Geometry check sheet. Reference: drawing and pictorial views, mm from the part's lowest x, y, z. A direction names the side the tool comes from. Coordinates: 2 decimals unless noted, no trailing zeros. Write each loop counter-clockwise with the first axis right and the second up, starting at its lowest first coordinate (ties: lowest second). Pieces come first, ordered by that corner, then holes. Notation, with made-up numbers: (11.5, 63.25) -> (55.5, 63.25) arc R34 cw to (55.5, 102.25) -> close; hole circle Ø5 at (-39, 69.5). An arc over 180 degrees is marked (long way). Answer in a Markdown table with one row per item.
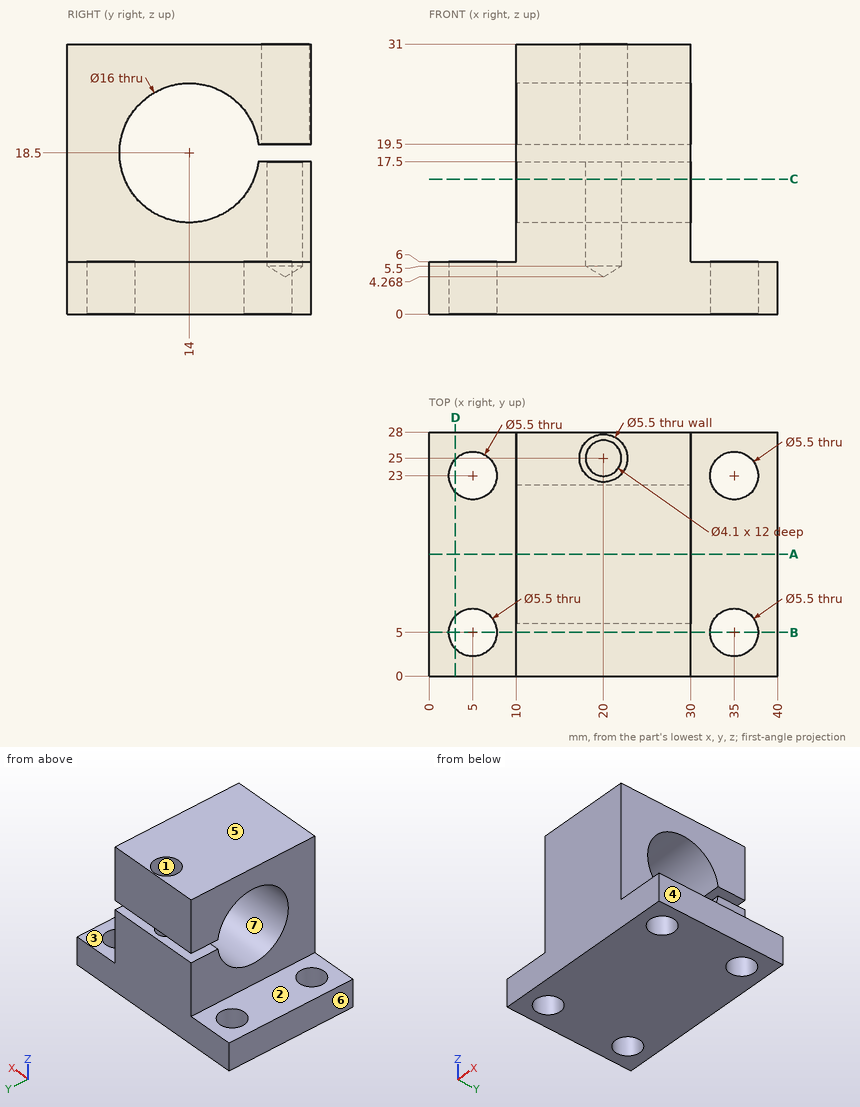
1. Section check C-C, the plane z = 15.5. Record the boundary of the cut face in (x, y), plus the area to 3 significant figures.
Geometry says:
| item | result |
|---|---|
| outline | (10, 0) -> (30, 0) -> (30, 6.58) -> (10, 6.58) -> close; (10, 21.42) -> (30, 21.42) -> (30, 28) -> (10, 28) -> close; hole circle Ø4.1 at (20, 25) |
| area | 250 mm^2 |
2. Tool access check on the marked faces 1, 2, 3 and 4. Record the directions out of +Z, -Z, +X, -X, +Y, -Y that give a thin tool (end or side, any length) a straight path to the whole face; none if there is none.
Geometry says:
| item | result |
|---|---|
| face 1 | +Z |
| face 2 | +Z, -X, +Y, -Y |
| face 3 | +Z, +X, +Y, -Y |
| face 4 | +Z, -Z, +X, +Y, -Y |
3. Depth check by flat-ended pin: P1, Ø6.5, axis at x = 35, y = 5, coming from the +Z side; P2, Ø12, axis at y = 23, z = 20.5, coming from the +X side; P3, Ø4.5, axis at x = 20, y = 25, coming from the +Z side. Enter the tip coordinate at first touch or a pass-through.
Geometry says:
| item | result |
|---|---|
| P1 | z = 6 |
| P2 | x = 30 |
| P3 | z = 17.5 |
4. Section check D-D, the plane x = 3. Record the boundary of the cut face in (y, z).
Geometry says:
| item | result |
|---|---|
| outline | (0, 0) -> (3.11, 0) -> (3.11, 6) -> (0, 6) -> close; (6.89, 0) -> (21.11, 0) -> (21.11, 6) -> (6.89, 6) -> close; (24.89, 0) -> (28, 0) -> (28, 6) -> (24.89, 6) -> close |
5. Thickness scan on line 1 (Y direction, x = 5, z = 1); line 2 (Z direction, x = 17.5, y = 26.5); line 3 (X direction, y = 24, z = 2.5). Record the ranges inside material, lowest first. Write a range as from..to.
Geometry says:
| item | result |
|---|---|
| line 1 | 0..2.25, 7.75..20.25, 25.75..28 |
| line 2 | 0..17.5, 19.5..31 |
| line 3 | 0..2.44, 7.56..32.44, 37.56..40 |
6. Section check B-B, the plane y = 5. Record the boundary of the cut face in (x, z), plus the area to 3 significant figures.
Geometry says:
| item | result |
|---|---|
| outline | (0, 0) -> (2.25, 0) -> (2.25, 6) -> (0, 6) -> close; (7.75, 0) -> (32.25, 0) -> (32.25, 6) -> (30, 6) -> (30, 31) -> (10, 31) -> (10, 6) -> (7.75, 6) -> close; (37.75, 0) -> (40, 0) -> (40, 6) -> (37.75, 6) -> close |
| area | 674 mm^2 |
7. Section check A-A, the plane y = 14. Record the boundary of the cut face in (x, z), plus the area to 3 significant figures.
Geometry says:
| item | result |
|---|---|
| outline | (0, 0) -> (40, 0) -> (40, 6) -> (30, 6) -> (30, 10.5) -> (10, 10.5) -> (10, 6) -> (0, 6) -> close; (10, 26.5) -> (30, 26.5) -> (30, 31) -> (10, 31) -> close |
| area | 420 mm^2 |
8. Mould release check, pull along Z, two halves, no side actions. Record for the marked faces 5, 6 and 7: released by +Z, released by -Z, zero draft, split by the parting line, or undercut.
Geometry says:
| item | result |
|---|---|
| face 5 | released by +Z |
| face 6 | zero draft |
| face 7 | undercut |
